Print and shaded views of the part. All mm, measured from the part's lowest x, y and z. A direction names the side the tool comes from. Round coordinates to 2 decimals unless told otherwise and drop trailing zeros. Loops run counter-clockwise (first coordinate to the right, second up) from the corner with the lowest first, then second, coordinate; pieces in that order, holes last. Notation, with made-up numbers: (16, -36.5) -> (46, -36.5) arc R25 ccw to (46, -5.5) -> close; hole circle Ø7 at (78, -7.75). An arc over 180 degrees is marked (long way). Use a Markdown table: item, result.
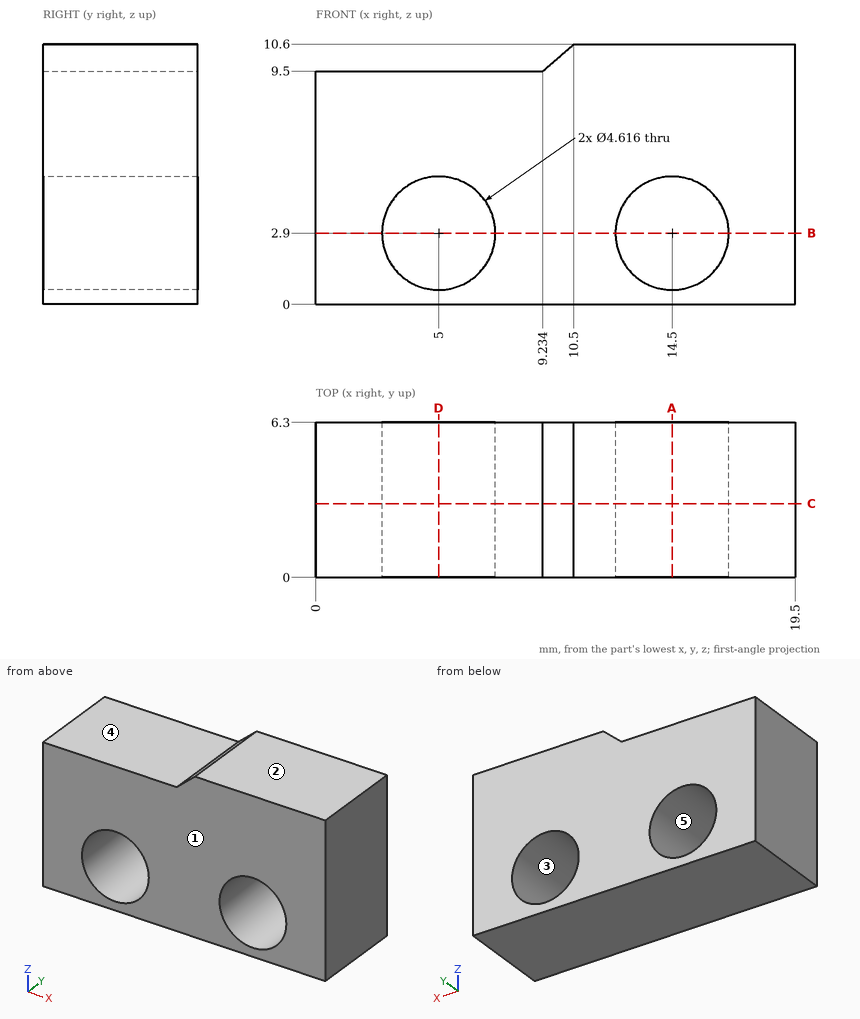
Q1. Pull direction Z, two halves, no side cores. Call the marked faces 1, 2 and 3: released by +Z, released by -Z, zero draft, split by the parting line, or undercut.
Results list:
| item | result |
|---|---|
| face 1 | zero draft |
| face 2 | released by +Z |
| face 3 | undercut |
Q2. Tool access for the marked faces 4 and 5: list every direction of +Z, -Z, +X, -X, +Y, -Y with a clear straight run to the whole face (end or side of a thin tool).
Results list:
| item | result |
|---|---|
| face 4 | +Z, -X, +Y, -Y |
| face 5 | +Y, -Y |
Q3. Band-saw the part on D-D, the plane x = 5. Give the cut face in (y, z).
Results list:
| item | result |
|---|---|
| outline | (0, 0) -> (6.3, 0) -> (6.3, 0.59) -> (0, 0.59) -> close; (0, 5.21) -> (6.3, 5.21) -> (6.3, 9.5) -> (0, 9.5) -> close |
Q4. Band-saw the part on C-C, the plane y = 3. Give the cut face in (x, z) (1 decimal), plus the area to 3 significant figures.
Results list:
| item | result |
|---|---|
| outline | (0, 0) -> (19.5, 0) -> (19.5, 10.6) -> (10.5, 10.6) -> (9.2, 9.5) -> (0, 9.5) -> close; hole circle Ø4.6 at (5, 2.9); hole circle Ø4.6 at (14.5, 2.9) |
| area | 162 mm² |
Q5. Band-saw the part on A-A, the plane x = 14.5. Give the cut face in (y, z).
Results list:
| item | result |
|---|---|
| outline | (0, 0) -> (6.3, 0) -> (6.3, 0.59) -> (0, 0.59) -> close; (0, 5.21) -> (6.3, 5.21) -> (6.3, 10.6) -> (0, 10.6) -> close |
Q6. Drill centre lines: L1, parallel to X at y = 3.5, z = 3 (1 decimal); L2, parallel to Z at x = 5, y = 3; L3, parallel to X at y = 1.25, z = 2 (1 decimal). Where is each one in solid material? Low to high. Write a range as from..to.
Results list:
| item | result |
|---|---|
| L1 | x = 0..2.7, 7.3..12.2, 16.8..19.5 |
| L2 | z = 0..0.59, 5.21..9.5 |
| L3 | x = 0..2.9, 7.1..12.4, 16.6..19.5 |
Q7. Flat gauge pins, fed straight in: pin 1 (3.5 mm diameter, centred on x = 14.5, z = 2.9, fed in from -Y); pin 2 (1 mm diameter, centred on x = 4.5, y = 1, fed in from +Z). Where does each tip first touch, or does it go through?
Results list:
| item | result |
|---|---|
| pin 1 | passes through |
| pin 2 | stops at z = 9.5 |
Q8. Band-saw the part on B-B, the plane z = 2.9. Give the cut face in (x, y).
Results list:
| item | result |
|---|---|
| outline | (0, 0) -> (2.69, 0) -> (2.69, 6.3) -> (0, 6.3) -> close; (7.31, 0) -> (12.19, 0) -> (12.19, 6.3) -> (7.31, 6.3) -> close; (16.81, 0) -> (19.5, 0) -> (19.5, 6.3) -> (16.81, 6.3) -> close |
